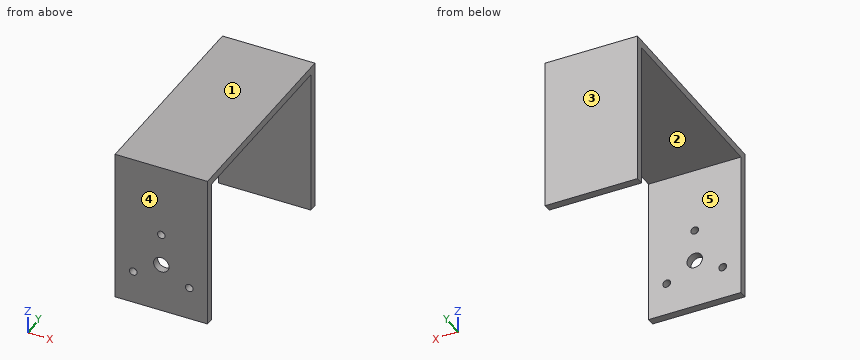
from build123d import *

# Parameters (mm, degrees)
SKETCH1_W           = 60
SKETCH1_H           = 100
BOSS_EXTRUDE1_DEPTH = 5
SKETCH2_W           = 60
SKETCH2_H           = 5
BOSS_EXTRUDE2_DEPTH = 130
SKETCH3_W           = 60
SKETCH3_H           = 5
BOSS_EXTRUDE3_DEPTH = 55
SKETCH9_W           = 60
SKETCH9_H           = 40
CUT_EXTRUDE1_DEPTH  = 55
SKETCH11_W          = 60
SKETCH11_H          = 5
BOSS_EXTRUDE4_DEPTH = 40
SKETCH12_W          = 60
SKETCH12_H          = 5
BOSS_EXTRUDE5_DEPTH = 40
SKETCH13_R          = 5
CUT_EXTRUDE2_DEPTH  = 40
SKETCH14_R          = 2.5
CUT_EXTRUDE3_DEPTH  = 40


with BuildPart() as part:
    # Sketch1 → Boss-Extrude1 (new body)
    with BuildSketch(Plane(origin=(0, 0, 0), x_dir=(1, 0, 0), z_dir=(0, 1, 0))):
        with Locations((-30, 50)):
            Rectangle(SKETCH1_W, SKETCH1_H)
    extrude(amount=BOSS_EXTRUDE1_DEPTH)

    # Sketch2 → Boss-Extrude2 (add)
    with BuildSketch(Plane(origin=(0, 5, 0), x_dir=(1, 0, 0), z_dir=(0, 1, 0))):
        with Locations((-30, 2.5)):
            Rectangle(SKETCH2_W, SKETCH2_H)
    extrude(amount=BOSS_EXTRUDE2_DEPTH)

    # Sketch3 → Boss-Extrude3 (add)
    with BuildSketch(Plane(origin=(0, 0, -5), x_dir=(-1, 0, 0), z_dir=(0, 0, -1))):
        with Locations((30, 132.5)):
            Rectangle(SKETCH3_W, SKETCH3_H)
    extrude(amount=BOSS_EXTRUDE3_DEPTH)

    # Sketch9 → Cut-Extrude1 (cut)
    with BuildSketch(Plane(origin=(0, 0, 0), x_dir=(-1, 0, 0), z_dir=(0, -1, 0))):
        with Locations((30, 80)):
            Rectangle(SKETCH9_W, SKETCH9_H)
    extrude(amount=-CUT_EXTRUDE1_DEPTH, mode=Mode.SUBTRACT)

    # Sketch11 → Boss-Extrude4 (add)
    with BuildSketch(Plane(origin=(0, 0, -60), x_dir=(-1, 0, 0), z_dir=(0, 0, -1))):
        with Locations((30, 132.5)):
            Rectangle(SKETCH11_W, SKETCH11_H)
    extrude(amount=BOSS_EXTRUDE4_DEPTH)

    # Sketch12 → Boss-Extrude5 (add)
    with BuildSketch(Plane(origin=(0, 0, -60), x_dir=(-1, 0, 0), z_dir=(0, 0, -1))):
        with Locations((30, 2.5)):
            Rectangle(SKETCH12_W, SKETCH12_H)
    extrude(amount=BOSS_EXTRUDE5_DEPTH)

    # Sketch13 → Cut-Extrude2 (cut)
    with BuildSketch(Plane.XZ):
        with Locations((-30, -68)):
            Circle(SKETCH13_R)
    extrude(amount=-CUT_EXTRUDE2_DEPTH, mode=Mode.SUBTRACT)

    # Sketch14 → Cut-Extrude3 (cut)
    with BuildSketch(Plane.XZ):
        with Locations((-30, -47)):
            Circle(SKETCH14_R)
        with Locations((-48.186533479, -78.5)):
            Circle(SKETCH14_R)
        with Locations((-11.813466521, -78.5)):
            Circle(SKETCH14_R)
    extrude(amount=-CUT_EXTRUDE3_DEPTH, mode=Mode.SUBTRACT)


solid = part.part
Read the model definition and answer for the solid it produces. Units are mm, in the model's axes. Face numbers are marked on the shaded views. A direction names the side the tool comes from. Coordinates: 2 decimals unless noted, no trailing zeros. Write each loop counter-clockwise with the first axis right and the second up, starting at its lowest first coordinate (ties: lowest second). Pieces come first, ordered by that corner, then holes. Notation, with made-up numbers: M -15.75,-3.5 L 21.25,-3.5 A22 cw 21.25,10.5 Z; hole C 26.5,-38 d2. An arc over 180 degrees is marked long. Use a Markdown table: item, result.
Q1. Each of these flat-tipped pins is pushed along its axis until it touches: pin 1 Ø4.5 at (x, z) = (-11.81, -78.5) entering from -Y; pin 2 Ø4 at (x, y) = (-24, 76.5) entering from -Z. Where does it stop, or does it pass through?
Answer block:
| item | result |
|---|---|
| pin 1 | stops at y = 130 |
| pin 2 | stops at z = -5 |
Q2. Which of the six approach directions +Z, -Z, +X, -X, +Y, -Y give full straight-line access (tool end or side, diameter ignored) to the marked faces 1 and 2?
Answer block:
| item | result |
|---|---|
| face 1 | +Z, +X, -X, +Y, -Y |
| face 2 | -Z, +X, -X |
Q3. The part is cut by section D-D, the plane z = -78.5. Write down the section's boundary in (x, y).
Answer block:
| item | result |
|---|---|
| outline | M -60,0 L -50.69,0 L -50.69,5 L -60,5 Z; M -60,130 L 0,130 L 0,135 L -60,135 Z; M -45.69,0 L -14.31,0 L -14.31,5 L -45.69,5 Z; M -9.31,0 L 0,0 L 0,5 L -9.31,5 Z |
Q4. The part is cut by section B-B, the plane x = -30. Write down the section's boundary in (y, z), then the cut area to 3 significant figures.
Answer block:
| item | result |
|---|---|
| outline | M 0,-100 L 5,-100 L 5,-73 L 0,-73 Z; M 0,-63 L 5,-63 L 5,-49.5 L 0,-49.5 Z; M 0,-44.5 L 5,-44.5 L 5,-5 L 130,-5 L 130,-100 L 135,-100 L 135,0 L 0,0 Z |
| area | 1,550 mm2 |
Q5. Determine the mould class of the marked faces 3, 4 and 5 for opening direction Y: released by +Y, released by -Y, zero draft, split by the parting line, or undercut.
Answer block:
| item | result |
|---|---|
| face 3 | released by +Y |
| face 4 | released by -Y |
| face 5 | undercut |
Q6. The part is cut by section C-C, the plane z = -24.5. Write down the section's boundary in (x, y).
Answer block:
| item | result |
|---|---|
| outline | M -60,0 L 0,0 L 0,5 L -60,5 Z; M -60,130 L 0,130 L 0,135 L -60,135 Z |
Q7. Straight lines are drawn through the part: L1, parallel to Z at x = -30, y = 1.85; L2, parallel to Y at x = -45, z = -70; L3, parallel to Z at x = -6, y = 121. For each, find the intervals that lie inside material, in ascending order. Write a range as [from, to].
Answer block:
| item | result |
|---|---|
| L1 | z = [-100, -73], [-63, -49.5], [-44.5, 0] |
| L2 | y = [0, 5], [130, 135] |
| L3 | z = [-5, 0] |
Q8. The part is cut by section A-A, the plane z = -47. Write down the section's boundary in (x, y), then the cut area to 3 significant figures.
Answer block:
| item | result |
|---|---|
| outline | M -60,0 L -32.5,0 L -32.5,5 L -60,5 Z; M -60,130 L 0,130 L 0,135 L -60,135 Z; M -27.5,0 L 0,0 L 0,5 L -27.5,5 Z |
| area | 575 mm2 |
